```python
from build123d import *

# Parameters (mm, degrees)
SKETCH1_R           = 1.6
BOSS_EXTRUDE1_DEPTH = 4
CUT_EXTRUDE7_DEPTH  = 1
CUT_EXTRUDE8_DEPTH  = 1.5
SKETCH8_R           = 4
BOSS_EXTRUDE5_DEPTH = 1.5
SKETCH13_R          = 1.5
CUT_EXTRUDE12_DEPTH = 17.5
CIRPATTERN2_COUNT   = 4
FILLET2_R           = 2
FILLET3_R           = 30


with BuildPart() as part:
    # Sketch1 → Boss-Extrude1 (new body)
    with BuildSketch(Plane.XY):
        Polygon((12.5, 35), (-12.5, 35), (-23.334523779, 36.062445841), (-36.062445841, 23.334523779), (-35, 12.5), (-35, -12.5), (-36.062445841, -23.334523779), (-23.334523779, -36.062445841), (-12.5, -35), (12.5, -35), (23.334523779, -36.062445841), (36.062445841, -23.334523779), (35, -12.5), (35, 12.5), (36.062445841, 23.334523779), (23.334523779, 36.062445841), align=None)
        with Locations((31.112698372, 22.627416998)):
            Circle(SKETCH1_R, mode=Mode.SUBTRACT)
        with Locations((22.627416998, 31.112698372)):
            Circle(SKETCH1_R, mode=Mode.SUBTRACT)
        with Locations((22.627416998, -31.112698372)):
            Circle(SKETCH1_R, mode=Mode.SUBTRACT)
        with Locations((31.112698372, -22.627416998)):
            Circle(SKETCH1_R, mode=Mode.SUBTRACT)
        with Locations((-31.112698372, -22.627416998)):
            Circle(SKETCH1_R, mode=Mode.SUBTRACT)
        with Locations((-22.627416998, -31.112698372)):
            Circle(SKETCH1_R, mode=Mode.SUBTRACT)
        with Locations((-22.627416998, 31.112698372)):
            Circle(SKETCH1_R, mode=Mode.SUBTRACT)
        with Locations((-31.112698372, 22.627416998)):
            Circle(SKETCH1_R, mode=Mode.SUBTRACT)
    extrude(amount=BOSS_EXTRUDE1_DEPTH)

    # 3DSketch1 → Cut-Extrude7 (cut, symmetric)
    with BuildSketch(Plane(origin=(-17.522554566, 30.250476628, 0.3336629), x_dir=(0.5012316605773316, -0.8653131354803826, 0), z_dir=(0, 0, -1))):
        Polygon((0, 0), (17.565718245, -30.324993267), (34.958993903, -34.958993903), (65.28398717, -17.393275658), (69.917987806, 0), (52.352269561, 30.324993267), (34.958993903, 34.958993903), (4.634000637, 17.393275658), align=None)
    extrude(amount=CUT_EXTRUDE7_DEPTH, both=True, mode=Mode.SUBTRACT)

    # Sketch7 → Cut-Extrude8 (cut)
    with BuildSketch(Plane(origin=(0, 0, 1.3336629), x_dir=(-1, 0, 0), z_dir=(0, 0, -1))):
        with BuildLine():
            Line((-15, -4.506640856), (-15, 4.506640856))
            ThreePointArc((-15, 4.506640856), (-15.314344635, 5.843523522), (-16.191503508, 6.900244925))
            Line((-16.191503508, 6.900244925), (-25.441980135, 13.889477085))
            ThreePointArc((-25.441980135, 13.889477085), (-28.587359293, 14.181528381), (-30.250476628, 11.495873016))
            Line((-30.250476628, 11.495873016), (-30.250476628, -11.495873016))
            ThreePointArc((-30.250476628, -11.495873016), (-28.587359293, -14.181528381), (-25.441980135, -13.889477085))
            Line((-25.441980135, -13.889477085), (-16.191503508, -6.900244925))
            ThreePointArc((-16.191503508, -6.900244925), (-15.314344635, -5.843523522), (-15, -4.506640856))
        make_face()
        with BuildLine():
            Line((13.889477085, 25.441980135), (6.900244925, 16.191503508))
            ThreePointArc((6.900244925, 16.191503508), (5.843523522, 15.314344635), (4.506640856, 15))
            Line((4.506640856, 15), (-4.506640856, 15))
            ThreePointArc((-4.506640856, 15), (-5.843523522, 15.314344635), (-6.900244925, 16.191503508))
            Line((-6.900244925, 16.191503508), (-13.889477085, 25.441980135))
            ThreePointArc((-13.889477085, 25.441980135), (-14.181528381, 28.587359293), (-11.495873016, 30.250476628))
            Line((-11.495873016, 30.250476628), (11.495873016, 30.250476628))
            ThreePointArc((11.495873016, 30.250476628), (14.181528381, 28.587359293), (13.889477085, 25.441980135))
        make_face()
        with BuildLine():
            Line((25.441980135, -13.889477085), (16.191503508, -6.900244925))
            ThreePointArc((16.191503508, -6.900244925), (15.314344635, -5.843523522), (15, -4.506640856))
            Line((15, -4.506640856), (15, 4.506640856))
            ThreePointArc((15, 4.506640856), (15.314344635, 5.843523522), (16.191503508, 6.900244925))
            Line((16.191503508, 6.900244925), (25.441980135, 13.889477085))
            ThreePointArc((25.441980135, 13.889477085), (28.587359293, 14.181528381), (30.250476628, 11.495873016))
            Line((30.250476628, 11.495873016), (30.250476628, -11.495873016))
            ThreePointArc((30.250476628, -11.495873016), (28.587359293, -14.181528381), (25.441980135, -13.889477085))
        make_face()
        with BuildLine():
            Line((-13.889477085, -25.441980135), (-6.900244925, -16.191503508))
            ThreePointArc((-6.900244925, -16.191503508), (-5.843523522, -15.314344635), (-4.506640856, -15))
            Line((-4.506640856, -15), (4.506640856, -15))
            ThreePointArc((4.506640856, -15), (5.843523522, -15.314344635), (6.900244925, -16.191503508))
            Line((6.900244925, -16.191503508), (13.889477085, -25.441980135))
            ThreePointArc((13.889477085, -25.441980135), (14.181528381, -28.587359293), (11.495873016, -30.250476628))
            Line((11.495873016, -30.250476628), (-11.495873016, -30.250476628))
            ThreePointArc((-11.495873016, -30.250476628), (-14.181528381, -28.587359293), (-13.889477085, -25.441980135))
        make_face()
    extrude(amount=-CUT_EXTRUDE8_DEPTH, mode=Mode.SUBTRACT)

    # Sketch8 → Boss-Extrude5 (add)
    with BuildSketch(Plane(origin=(0, 0, 1.3336629), x_dir=(-1, 0, 0), z_dir=(0, 0, -1))):
        with Locations((15.25, 15.25)):
            Circle(SKETCH8_R)
    boss_extrude5 = extrude(amount=BOSS_EXTRUDE5_DEPTH)

    # Sketch13 → Cut-Extrude12 (cut)
    with BuildSketch(Plane(origin=(0, 0, -0.1663371), x_dir=(-1, 0, 0), z_dir=(0, 0, -1))):
        with Locations((15.25, 15.25)):
            Circle(SKETCH13_R)
    cut_extrude12 = extrude(amount=-CUT_EXTRUDE12_DEPTH, mode=Mode.SUBTRACT)

    # CirPattern2: Boss-Extrude5, Cut-Extrude12 ×4 about axis
    cirpattern2_axis = Axis((0, 0, 0), (0, 0, 1))
    add([boss_extrude5.rotate(cirpattern2_axis, i * 360 / CIRPATTERN2_COUNT) for i in range(1, CIRPATTERN2_COUNT)])
    add([cut_extrude12.rotate(cirpattern2_axis, i * 360 / CIRPATTERN2_COUNT) for i in range(1, CIRPATTERN2_COUNT)], mode=Mode.SUBTRACT)

    # Fillet2
    # the kernel refuses this fillet: 2 mm, written as the material it adds along each edge
    with BuildSketch(Plane(origin=(-15.25, 15.25, 1.3336629), x_dir=(-1, 0, 0), z_dir=(0, -1, 0))) as fillet2_piece_1:
        with BuildLine():
            CenterArc((5.936491673, 2), FILLET2_R, 194.477512186, 75.522487814)
            Line((4, 1.5), (3.961270167, 1.49))
            ThreePointArc((3.961270167, 1.49), (3.96, 0.75), (3.96, 0))
            Line((3.96, 0), (4, -0.04))
            Line((4, -0.04), (5.936491673, -0.04))
            Line((5.936491673, -0.04), (5.936491673, 0))
        make_face()
    revolve(axis=Axis((-15.25, 15.25, 1.3336629), (0, 0, -1)))
    with BuildSketch(Plane(origin=(-15.25, -15.25, 1.3336629), x_dir=(0, -1, 0), z_dir=(1, 0, 0))) as fillet2_piece_2:
        with BuildLine():
            CenterArc((5.936491673, 2), FILLET2_R, 194.477512186, 75.522487814)
            Line((4, 1.5), (3.961270167, 1.49))
            ThreePointArc((3.961270167, 1.49), (3.96, 0.75), (3.96, 0))
            Line((3.96, 0), (4, -0.04))
            Line((4, -0.04), (5.936491673, -0.04))
            Line((5.936491673, -0.04), (5.936491673, 0))
        make_face()
    revolve(axis=Axis((-15.25, -15.25, 1.3336629), (0, 0, -1)))
    with BuildSketch(Plane(origin=(15.25, -15.25, 1.3336629), x_dir=(1, 0, 0), z_dir=(0, 1, 0))) as fillet2_piece_3:
        with BuildLine():
            CenterArc((5.936491673, 2), FILLET2_R, 194.477512186, 75.522487814)
            Line((4, 1.5), (3.961270167, 1.49))
            ThreePointArc((3.961270167, 1.49), (3.96, 0.75), (3.96, 0))
            Line((3.96, 0), (4, -0.04))
            Line((4, -0.04), (5.936491673, -0.04))
            Line((5.936491673, -0.04), (5.936491673, 0))
        make_face()
    revolve(axis=Axis((15.25, -15.25, 1.3336629), (0, 0, -1)))
    with BuildSketch(Plane(origin=(15.25, 15.25, 1.3336629), x_dir=(0, 1, 0), z_dir=(-1, 0, 0))) as fillet2_piece_4:
        with BuildLine():
            CenterArc((5.936491673, 2), FILLET2_R, 194.477512186, 75.522487814)
            Line((4, 1.5), (3.961270167, 1.49))
            ThreePointArc((3.961270167, 1.49), (3.96, 0.75), (3.96, 0))
            Line((3.96, 0), (4, -0.04))
            Line((4, -0.04), (5.936491673, -0.04))
            Line((5.936491673, -0.04), (5.936491673, 0))
        make_face()
    revolve(axis=Axis((15.25, 15.25, 1.3336629), (0, 0, -1)))

    # Fillet3
    # the kernel refuses this fillet: 30 mm, written as the material it adds along each edge
    with BuildSketch(Plane(origin=(-12.5, 35, 0), x_dir=(1, 0, 0), z_dir=(0, 0, 1)), Plane(origin=(-12.5, -35, 0), x_dir=(-0.995226405289247, -0.09759304388655768, 0), z_dir=(0, 0, 1)), Plane(origin=(-35, -12.5, 0), x_dir=(0, 1, 0), z_dir=(0, 0, 1)), Plane(origin=(-35, 12.5, 0), x_dir=(-0.09759304388655696, 0.9952264052892469, 0), z_dir=(0, 0, 1))) as fillet3_piece_1:
        with BuildLine():
            CenterArc((FILLET3_R * 0.0489132680019, FILLET3_R), FILLET3_R, 264.399415997, 5.600584003)
            Line((-FILLET3_R * 0.0486797758845, FILLET3_R * 0.00477359471074), (0, 0))
            Line((0, 0), (FILLET3_R * 0.0489132680019, 0))
        make_face()
    extrude(amount=4)
    with BuildSketch(Plane(origin=(12.5, 35, 0), x_dir=(-1, 0, 0), z_dir=(0, 0, 1)), Plane(origin=(35, 12.5, 0), x_dir=(0.09759304388646403, 0.9952264052892561, 0), z_dir=(0, 0, 1)), Plane(origin=(35, -12.5, 0), x_dir=(0, 1, 0), z_dir=(0, 0, 1)), Plane(origin=(12.5, -35, 0), x_dir=(0.9952264052892558, -0.09759304388646729, 0), z_dir=(0, 0, 1))) as fillet3_piece_2:
        with BuildLine():
            CenterArc((FILLET3_R * 0.048913268002, -FILLET3_R), FILLET3_R, 90, 5.600584003)
            Line((-FILLET3_R * 0.0486797758846, -FILLET3_R * 0.00477359471075), (0, 0))
            Line((0, 0), (FILLET3_R * 0.048913268002, 0))
        make_face()
    extrude(amount=4)


solid = part.part
```
Could you check a few things on this model? Use its own coordinates, in mm. A direction names the side the tool comes from. Coordinates: 2 decimals unless noted, no trailing zeros. Loops run counter-clockwise (first coordinate to the right, second up) from the corner with the lowest first, then second, coordinate; pieces in that order, holes last. Notation, with made-up numbers: M -29.5,78 L -13.5,78 A24 cw -13.5,89 Z; hole C 37.25,-27 d6. An arc over 180 degrees is marked long. Put each result on its own line as item: value. Start each with the question number.
(1) Will these pins go through, and if not, where does the flat tip stop? P1, Ø1.7, axis at y = 1.5, z = 2, coming from the -X side; P2, Ø1.2, axis at x = 0.5, z = 1.5, coming from the -Y side; P3, Ø1.7, axis at x = -3, z = 2, coming from the +Y side; P4, Ø3, axis at x = -22.63, y = 31.11, coming from the +Z side.
(2) Thinking about a two-plate mould opening in Y: for faces 1 (the face through (-15.2, 13.5, -0.166)), 2 (the face through (10.346, 20.752, 2.073)), 3 (the face through (-18.6, 35.6, 2)), which applies, pulls with the +Y half, pulls with the -Y half, needs draft (parallel to the pull), parting line crosses it, or undercut?
(3) I need wall thicknesses on line 1 (X direction, y = -1.5, z = 2.75); line 2 (X direction, y = -15.25, z = 2.7); line 3 (Y direction, x = 31, z = 0.8). Which ranges of each line are inside material? Lowest first, please. Write a range as from..to.
(4) For faces 4 (the face through (14.2, 28.55, 2.07)), 5 (the face through (35, 0, 2)), 6 (the face through (-35.61, 18.71, 1.97)), which set-ups out of +Z, -Z, +X, -X, +Y, -Y let a thin tool reach every point of the face, with its end or its side?
(5) Suppose I cut it at A-A on x = -27. Please give me the cut outline in (y, z), then the cut area to 3 significant figures.
Solutions:
1. P1: stops at x = -35
1. P2: stops at y = -35
1. P3: stops at y = 35
1. P4: passes through
2. face 1: needs draft
2. face 2: undercut
2. face 3: pulls with the +Y half
3. line 1: x = -35..-30.25, -15..15, 30.25..35
3. line 2: x = -35.27..-16.75, -13.75..-5.71, 5.71..13.75, 16.75..35.27
3. line 3: y = -28.4..-24.22, -21.03..21.03, 24.22..28.4
4. face 4: -Z
4. face 5: +Z, -Z, +X
4. face 6: +Z, -Z, -X
5. outline: M -32.4,0 L -20.77,0 L -20.77,1.33 L -14.49,1.33 L -14.49,2.83 L 14.49,2.83 L 14.49,1.33 L 20.77,1.33 L 20.77,0 L 32.4,0 L 32.4,4 L -32.4,4 Z
5. area: 160 mm2
